The model under review builds one solid part; all positions refer to its coordinate system, in mm. A direction names the side the tool comes from. Give positions to 0.01 mm unless a question says otherwise; leave off trailing zeros. Write each loop counter-clockwise with the first axis right and the second up, starting at its lowest first coordinate (ties: lowest second). Pieces come first, ordered by that corner, then holes. Notation, with made-up numbers: (-20.5, 75.5) - (18.5, 75.5) arc R32 ccw to (18.5, 102.5) - close; hole circle Ø11 at (-16, -5). An arc over 180 degrees is marked (long way). Write item = value, one per line.
```python
from build123d import *

# Parameters (mm, degrees)
F0_R     = 2.75
F0_R_2   = 6.35
F1_DEPTH = 12.7


with BuildPart() as f1:
    # F0 (on Top) → F1 (new body)
    with BuildSketch(Plane.XY):
        with BuildLine():
            Line((4.5, 10.85), (4.5, 21.5))
            ThreePointArc((4.5, 21.5), (0, 26), (-4.5, 21.5))
            Line((-4.5, 21.5), (-4.5, 10.85))
            ThreePointArc((-4.5, 10.85), (-6.359872, 6.359872), (-10.85, 4.5))
            Line((-10.85, 4.5), (-21.5, 4.5))
            ThreePointArc((-21.5, 4.5), (-26, 0), (-21.5, -4.5))
            Line((-21.5, -4.5), (-10.85, -4.5))
            ThreePointArc((-10.85, -4.5), (-6.359872, -6.359872), (-4.5, -10.85))
            Line((-4.5, -10.85), (-4.5, -21.5))
            ThreePointArc((-4.5, -21.5), (0, -26), (4.5, -21.5))
            Line((4.5, -21.5), (4.5, -10.85))
            ThreePointArc((4.5, -10.85), (6.359872, -6.359872), (10.85, -4.5))
            Line((10.85, -4.5), (21.5, -4.5))
            ThreePointArc((21.5, -4.5), (26, 0), (21.5, 4.5))
            Line((21.5, 4.5), (10.85, 4.5))
            ThreePointArc((10.85, 4.5), (6.359872, 6.359872), (4.5, 10.85))
        make_face()
        with Locations((0, -21.5)):
            Circle(F0_R, mode=Mode.SUBTRACT)
        with Locations((-21.5, 0)):
            Circle(F0_R, mode=Mode.SUBTRACT)
        Circle(F0_R_2, mode=Mode.SUBTRACT)
        with Locations((21.5, 0)):
            Circle(F0_R, mode=Mode.SUBTRACT)
        with Locations((0, 21.5)):
            Circle(F0_R, mode=Mode.SUBTRACT)
    extrude(amount=F1_DEPTH)


solid = f1.part
```
1. Draft analysis for pull direction X (two halves, no side actions). For faces 5 (the cylindrical face through (-6.41, -6.31, 6.26)), 6 (the cylindrical face through (26, 0, 6)), 7 (the cylindrical face through (-0.358, -18.773, 6.261)), 8 (the flat face through (-4, 6, 12.7)), state which applies: +X half, -X half, draft (parallel to the pull), parting line (faces both ways), or undercut.
Findings below:
face_5 = -X half
face_6 = +X half
face_7 = undercut
face_8 = draft
2. Take a section at B-B on z = 6.5. Give the boundary of the cut face in (x, y), and give its area (3 significant figures).
Findings below:
outline = (-21.5, -4.5) - (-10.85, -4.5) arc R6.35 cw to (-4.5, -10.85) - (-4.5, -21.5) arc R4.5 ccw to (4.5, -21.5) - (4.5, -10.85) arc R6.35 cw to (10.85, -4.5) - (21.5, -4.5) arc R4.5 ccw to (21.5, 4.5) - (10.85, 4.5) arc R6.35 cw to (4.5, 10.85) - (4.5, 21.5) arc R4.5 ccw to (-4.5, 21.5) - (-4.5, 10.85) arc R6.35 cw to (-10.85, 4.5) - (-21.5, 4.5) arc R4.5 ccw to start; hole circle Ø5.5 at (-21.5, 0); hole circle Ø12.7 at (0, 0); hole circle Ø5.5 at (0, -21.5); hole circle Ø5.5 at (0, 21.5); hole circle Ø5.5 at (21.5, 0)
area = 633 mm²
3. Insertion check: P1, Ø9, axis at x = 0, y = 21.5, coming from the -Z side; P2, Ø3, axis at y = 14.5, z = 5.5, coming from the -X side; P3, Ø1.5, axis at x = -2.5, z = 7, coming from the -Y side; P4, Ø5, axis at x = -6, z = 2, coming from the +Y side. Each pin has a flat end and moves straight along its axis. Give the tip position at first contact, or say it passes through.
Findings below:
P1 = 0
P2 = -4.5
P3 = -25.65
P4 = 24.33
4. Machinability: for faces 1 (the flat face through (-4.5, -16, 6)), 2 (the flat face through (16, -4.5, 6)), 3 (the flat face through (-4.5, 16, 6)), 4 (the flat face through (16, 4.5, 6)), which of the approach directions +Z, -Z, +X, -X, +Y, -Y give a long, thin tool a straight path to every point of the face, cutting with its end or side? Answer none if there is none.
Findings below:
face_1 = +Z, -Z, -X, -Y
face_2 = +Z, -Z, +X, -Y
face_3 = +Z, -Z, -X, +Y
face_4 = +Z, -Z, +X, +Y
5. Take a section at A-A on x = 0. Give the boundary of the cut face in (y, z), and give its area (3 significant figures).
Findings below:
outline = (-26, 0) - (-24.25, 0) - (-24.25, 12.7) - (-26, 12.7) - close; (-18.75, 0) - (-6.35, 0) - (-6.35, 12.7) - (-18.75, 12.7) - close; (6.35, 0) - (18.75, 0) - (18.75, 12.7) - (6.35, 12.7) - close; (24.25, 0) - (26, 0) - (26, 12.7) - (24.25, 12.7) - close
area = 359 mm²
6. Take a section at D-D on y = -22.5. Give the boundary of the cut face in (x, z), and give its area (3 significant figures).
Findings below:
outline = (-4.39, 0) - (-2.56, 0) - (-2.56, 12.7) - (-4.39, 12.7) - close; (2.56, 0) - (4.39, 0) - (4.39, 12.7) - (2.56, 12.7) - close
area = 46.4 mm²
7. For line 1 (Y direction, x = 0, z = 3); line 2 (Y direction, x = -21.5, z = 5.75); line 3 (Y direction, x = 13.5, z = 4.5), list the stretches that pass through material, from the lowest coordinate up. Write a range as from..to.
Findings below:
line_1 = -26..-24.25, -18.75..-6.35, 6.35..18.75, 24.25..26
line_2 = -4.5..-2.75, 2.75..4.5
line_3 = -4.5..4.5
